```python
from build123d import *

# Parameters (mm, degrees)
SKETCH_R        = 1.8
PAD_DEPTH       = 7
SKETCH001_R     = 2.9
POCKET_DEPTH    = 3
SKETCH002_W     = 13.4
SKETCH002_H     = 5
PAD001_DEPTH    = 6
SKETCH005_R     = 1.8
POCKET002_DEPTH = 5
SKETCH009_W     = 8.2
SKETCH009_H     = 18
POCKET006_DEPTH = 3.6
POCKET003_DEPTH = 47.001
POCKET004_DEPTH = 5
POCKET005_DEPTH = 3.401
PAD002_DEPTH    = 2
FILLET_R        = 1.5


with BuildPart() as part:
    # Sketch → Pad (new body)
    with BuildSketch(Plane.XY):
        with BuildLine():
            Line((-21.5, 0), (-21.5, -5))
            Line((-21.5, -5), (-8.1, -5))
            Line((-8.1, -5), (-8.1, -18))
            ThreePointArc((-10.421049, -20.922161), (-8.750867, -19.865898), (-8.1, -18))
            Line((-10.421049, -20.922161), (-22.018426, -23.616758))
            ThreePointArc((-22.018426, -23.616758), (-25.108802, -29.835142), (-18.415416, -31.683738))
            Line((-7.079536, -23.730259), (-18.415416, -31.683738))
            ThreePointArc((-7.079536, -23.730259), (-4.889394, -21.2293), (-4.1, -18))
            Line((-4.1, -18), (-4.1, -25))
            Line((-4.1, -25), (4.1, -25))
            Line((4.1, -18), (4.1, -25))
            ThreePointArc((4.1, -18), (4.889394, -21.2293), (7.079536, -23.730259))
            Line((7.079536, -23.730259), (18.415416, -31.683738))
            ThreePointArc((18.415416, -31.683738), (25.108802, -29.835142), (22.018426, -23.616758))
            Line((10.421049, -20.922161), (22.018426, -23.616758))
            ThreePointArc((8.1, -18), (8.750867, -19.865898), (10.421049, -20.922161))
            Line((8.1, -5), (8.1, -18))
            Line((21.5, -5), (8.1, -5))
            Line((21.5, -5), (21.5, 0))
            Line((21.5, 0), (4.1, 0))
            Line((4.1, 0), (4.1, -7))
            Line((-4.1, -7), (4.1, -7))
            Line((-4.1, 0), (-4.1, -7))
            Line((-21.5, 0), (-4.1, 0))
        make_face()
        with Locations((-21, -28)):
            Circle(SKETCH_R, mode=Mode.SUBTRACT)
        with Locations((21, -28)):
            Circle(SKETCH_R, mode=Mode.SUBTRACT)
    extrude(amount=PAD_DEPTH)

    # Sketch001 (on Face28 of Pad) → Pocket (cut)
    with BuildSketch(Plane.XY.offset(7)):
        with Locations((-21, -28)):
            Circle(SKETCH001_R)
        with Locations((21, -28)):
            Circle(SKETCH001_R)
    extrude(amount=-POCKET_DEPTH, mode=Mode.SUBTRACT)

    # Sketch002 (on Face5 of Pocket) → Pad001 (join)
    with BuildSketch(Plane.XY.offset(7)):
        with Locations((14.8, -2.5)):
            Rectangle(SKETCH002_W, SKETCH002_H)
        with Locations((-14.8, -2.5)):
            Rectangle(SKETCH002_W, SKETCH002_H)
    extrude(amount=PAD001_DEPTH)

    # Sketch005 (on Face32 of Pad001) → Pocket002 (cut)
    with BuildSketch(Plane(origin=(0, 0, 0), x_dir=(-1, 0, 0), z_dir=(0, 1, 0))):
        with Locations((-16, 9)):
            Circle(SKETCH005_R)
        with Locations((16, 9)):
            Circle(SKETCH005_R)
    extrude(amount=-POCKET002_DEPTH, mode=Mode.SUBTRACT)

    # Sketch009 (on Face31 of Pocket002) → Pocket006 (cut)
    with BuildSketch(Plane.XY.offset(7)):
        with Locations((0, -16)):
            Rectangle(SKETCH009_W, SKETCH009_H)
    extrude(amount=-POCKET006_DEPTH, mode=Mode.SUBTRACT)

    # Sketch006 (on Face2 of Pocket006) → Pocket003 (cut, through all)
    with BuildSketch(Plane(origin=(-21.5, 0, 0), x_dir=(0, -1, 0), z_dir=(-1, 0, 0))):
        Polygon((5, 0), (0, 0), (0, 5), align=None)
    extrude(amount=-POCKET003_DEPTH, mode=Mode.SUBTRACT)

    # Sketch007 (on Face25 of Pocket003) → Pocket004 (cut)
    with BuildSketch(Plane.XZ.offset(5)):
        Polygon((-21.5, 0), (-21.5, 9), (-12.5, 0), align=None)
        Polygon((21.5, 0), (21.5, 9), (12.5, 0), align=None)
    extrude(amount=-POCKET004_DEPTH, mode=Mode.SUBTRACT)

    # Sketch008 (on Face27 of Pocket004) → Pocket005 (cut, through all)
    with BuildSketch(Plane.XY.offset(3.4)):
        with BuildLine():
            ThreePointArc((1.8, -14), (0, -12.2), (-1.8, -14))
            Line((-1.8, -14), (-1.8, -19))
            ThreePointArc((-1.8, -19), (0, -20.8), (1.8, -19))
            Line((1.8, -14), (1.8, -19))
        make_face()
    extrude(amount=-POCKET005_DEPTH, mode=Mode.SUBTRACT)

    # Sketch010 (on Face17 of Pocket005) → Pad002 (join)
    with BuildSketch(Plane.XZ.offset(25)):
        Polygon((-4.1, 4.9), (-5.1, 4.9), (-5.1, 0), (-4.1, 0), (-4.1, 3.4), (-3.7, 3.4), align=None)
        Polygon((4.1, 0), (5.1, 0), (5.1, 4.9), (4.1, 4.9), (3.7, 3.4), (4.1, 3.4), align=None)
    extrude(amount=-PAD002_DEPTH)

    # Fillet
    fillet_edges = [part.edges().sort_by_distance(p)[0] for p in [
        (-12.747476, -27.706999, 7),
        (12.747476, -27.706999, 7),
    ]]
    fillet(fillet_edges, radius=FILLET_R)


solid = part.part
```
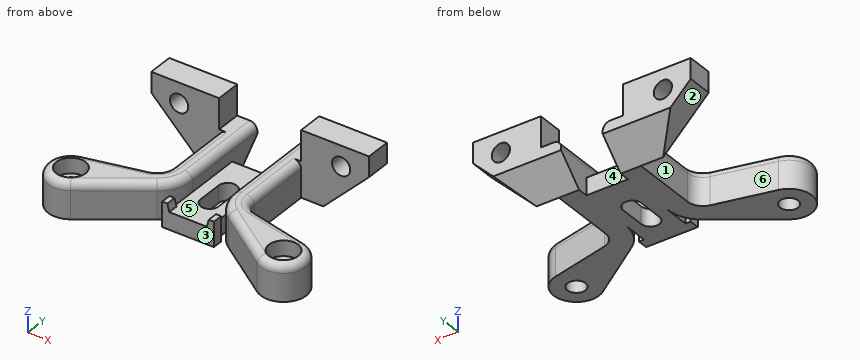
Check sheet for the modelled part. Datum: model origin and axes. Units: mm. Face numbers are marked on the shaded views. A direction names the side the tool comes from. Give positions to 0.01 mm unless a question says otherwise; leave off trailing zeros. Order: outer loops, then holes, each group sorted by start corner. A loop starts at its lowest first (then second) coordinate and runs counter-clockwise, first axis right, second up. Notation, with made-up numbers: M 89,-12.75 L 138,-12.75 A24 ccw 138,4.25 Z; hole C 7.5,53.5 d5. An arc over 180 degrees is marked long. Answer in a Markdown table with one row per item. Add a question column.
Q1. Sectioned sample at B-B, the plane y = -16. Record the boundary of the cut face in (x, z), and give its area (3 significant figures).
Q2. Sectioned sample at C-C, the plane x = 0. Record the boundary of the cut face in (y, z).
Q3. Access from +Z, -Z, +X, -X, +Y, -Y to the whole of each face (thin tool, end or side, straight path). Record for the marked faces 1, 2 and 3.
Q4. Sectioned sample at D-D, the plane z = 8. Record the boundary of the cut face in (x, y).
Q5. Sectioned sample at A-A, the plane y = -3. Record the boundary of the cut face in (x, z), and give its area (3 significant figures).
Q6. Release check for a two-part mould opening along Y. For the marked faces 4, 5 and 6 record: released by +Y, released by -Y, zero draft, split by the parting line, or undercut.
Q7. Thickness scan on L1, parallel to X at y = -15.5, z = 5; L2, parallel to X at y = -28, z = 1.3; L3, parallel to Y at x = -21, z = 2.4. Record the ranges inside material, lowest first.
Q8. Gauge pin test, flat ends, axial feed: pin 1 Ø6.5 at (x, z) = (12, 3.5) entering from -Y; pin 2 Ø1.5 at (x, z) = (4.5, 2.5) entering from +Y; pin 3 Ø1 at (x, y) = (5, -18.5) entering from +Z; pin 4 Ø2 at (x, y) = (14, -19.5) entering from +Z. Record the tip position at first contact, or that the pin passes through.
Verdict:
| question | item | result |
|---|---|---|
| 1 | outline | M -8.1,0 L -1.8,0 L -1.8,3.4 L -4.1,3.4 L -4.1,5.5 A1.5 ccw -5.6,7 L -6.6,7 A1.5 ccw -8.1,5.5 Z; M 1.8,0 L 8.1,0 L 8.1,5.5 A1.5 ccw 6.6,7 L 5.6,7 A1.5 ccw 4.1,5.5 L 4.1,3.4 L 1.8,3.4 Z |
| 1 | area | 69.7 mm² |
| 2 | outline | M -25,0 L -20.8,0 L -20.8,3.4 L -25,3.4 Z; M -12.2,0 L -7,0 L -7,3.4 L -12.2,3.4 Z |
| 3 | face 1 | +Z, -Z, -X |
| 3 | face 2 | -Z, -X, +Y |
| 3 | face 3 | +Z, -Z, -Y |
| 4 | outline | M -20.5,-5 L -17.5,-5 L -17.5,0 L -20.5,0 Z; M -14.5,-5 L -8.1,-5 L -8.1,0 L -14.5,0 Z; M 8.1,-5 L 14.5,-5 L 14.5,0 L 8.1,0 Z; M 17.5,-5 L 20.5,-5 L 20.5,0 L 17.5,0 Z |
| 5 | outline | M -21.5,9 L -14.5,2 L -4.1,2 L -4.1,5.5 A1.5 ccw -5.6,7 L -8.1,7 L -8.1,13 L -21.5,13 Z; M 4.1,2 L 14.5,2 L 21.5,9 L 21.5,13 L 8.1,13 L 8.1,7 L 5.6,7 A1.5 ccw 4.1,5.5 Z; hole C -16,9 d3.6; hole C 16,9 d3.6 |
| 5 | area | 264 mm² |
| 6 | face 4 | released by +Y |
| 6 | face 5 | zero draft |
| 6 | face 6 | undercut |
| 7 | L1 | -8.1 to -4.1, 4.1 to 8.1 |
| 7 | L2 | -25.5 to -22.8, -19.2 to -13.17, 13.17 to 19.2, 22.8 to 25.5 |
| 7 | L3 | -32.5 to -29.8, -26.2 to -23.38 |
| 8 | pin 1 | y = -29.46 |
| 8 | pin 2 | y = -1.75 |
| 8 | pin 3 | z = 7 |
| 8 | pin 4 | through |
